Read the model definition and answer for the solid it produces. Units are mm, in the model's axes. Give positions to 0.01 mm unless a question says otherwise; leave off trailing zeros. Write each loop counter-clockwise with the first axis right and the second up, starting at its lowest first coordinate (ties: lowest second). Pieces come first, ordered by that corner, then holes.
```python
from build123d import *

# Parameters (mm, degrees)
BOSS_EXTRUDE1_DEPTH = 600
SKETCH2_R           = 4
CUT_EXTRUDE1_DEPTH  = 26


with BuildPart() as part:
    # Sketch1 → Boss-Extrude1 (new body)
    with BuildSketch(Plane.XY):
        Polygon((-10, 0), (0, 0), (0, 17.5), (-7, 17.5), (-10, 14.5), (-10, 12.5), (-7.75, 10.25), (-7.75, 8.25), (-10, 6), align=None)
        Polygon((0, 17.5), (0, 0), (10, 0), (10, 6), (7.75, 8.25), (7.75, 10.25), (10, 12.5), (10, 14.5), (7, 17.5), align=None)
    extrude(amount=-BOSS_EXTRUDE1_DEPTH)

    # Sketch2 → Cut-Extrude1 (cut)
    with BuildSketch(Plane(origin=(0, 17.5, 0), x_dir=(1, 0, 0), z_dir=(0, 1, 0))):
        with Locations(Location((0, 30, 0), (0, 0, 270))):
            Circle(SKETCH2_R)
        with Locations(Location((0, 90, 0), (0, 0, 270))):
            Circle(SKETCH2_R)
        with Locations(Location((0, 150, 0), (0, 0, 270))):
            Circle(SKETCH2_R)
        with Locations(Location((0, 210, 0), (0, 0, 270))):
            Circle(SKETCH2_R)
        with Locations(Location((0, 270, 0), (0, 0, 270))):
            Circle(SKETCH2_R)
        with Locations(Location((0, 330, 0), (0, 0, 270))):
            Circle(SKETCH2_R)
        with Locations(Location((0, 390, 0), (0, 0, 270))):
            Circle(SKETCH2_R)
        with Locations(Location((0, 450, 0), (0, 0, 270))):
            Circle(SKETCH2_R)
        with Locations(Location((0, 510, 0), (0, 0, 270))):
            Circle(SKETCH2_R)
        with Locations(Location((0, 570, 0), (0, 0, 270))):
            Circle(SKETCH2_R)
    extrude(amount=-CUT_EXTRUDE1_DEPTH, mode=Mode.SUBTRACT)


solid = part.part
```
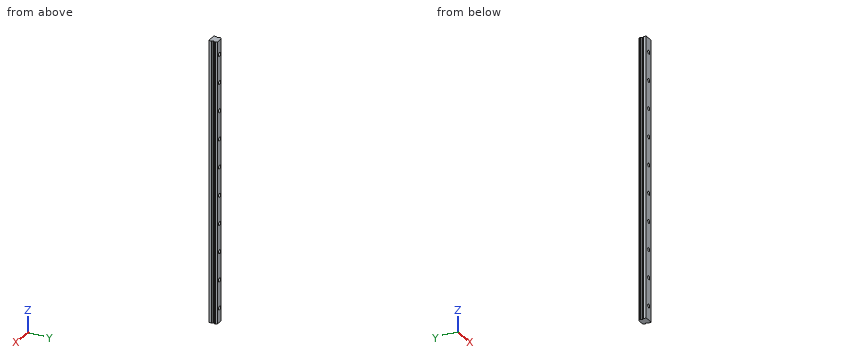
Item 1: Section A-A (z = -469.5) is taken. Write down the section's boundary in (x, y), and give its area (3 significant figures).
Result set:
outline: (-10, 0) - (10, 0) - (10, 6) - (7.75, 8.25) - (7.75, 10.25) - (10, 12.5) - (10, 14.5) - (7, 17.5) - (-7, 17.5) - (-10, 14.5) - (-10, 12.5) - (-7.75, 10.25) - (-7.75, 8.25) - (-10, 6) - close
area: 322 mm2
Item 2: Find the intervals of material crossed by line 1 along X through (y, z) = (13, -510); line 2 along X through (y, z) = (7, -89); line 3 along X through (y, z) = (9.25, -339.5), in increasing order.
Result set:
line 1: x = -10 to -4, 4 to 10
line 2: x = -9 to -3.87, 3.87 to 9
line 3: x = -7.75 to 7.75
Item 3: Each of these flat-tipped pins is pushed along its axis until it touches: pin 1 Ø1 at (y, z) = (9, -322) entering from -X; pin 2 Ø2 at (x, y) = (2.5, 7.5) entering from +Z; pin 3 Ø1.6 at (y, z) = (9.5, -231.5) entering from +X; pin 4 Ø3 at (y, z) = (9.5, -115.5) entering from -X. Where does it stop, or does it pass through?
Result set:
pin 1: stops at x = -7.75
pin 2: stops at z = 0
pin 3: stops at x = 7.8
pin 4: stops at x = -8.5
